from build123d import *

# Parameters (mm, degrees)
F0_W      = 59
F0_H      = 46
F1_DEPTH  = 32
F2_W      = 10
F2_H      = 6
F3_DEPTH  = 59
F4_W      = 33
F4_H      = 10
F5_DEPTH  = 23
F6_DEPTH  = 32
F8_DEPTH  = 26
F9_W      = 16
F9_H      = 12
F9_W_2    = 22
F10_DEPTH = 26
F12_DEPTH = 2
F13_R     = 2.5
F14_DEPTH = 25


with BuildPart() as f1:
    # F0 (on Top) → F1 (new body)
    with BuildSketch(Plane.XY):
        Rectangle(F0_W, F0_H)
    extrude(amount=F1_DEPTH)

    # F2 (on face) → F3 (cut)
    with BuildSketch(Plane.YZ.offset(29.5)):
        with Locations((0, 3)):
            Rectangle(F2_W, F2_H)
    extrude(amount=-F3_DEPTH, mode=Mode.SUBTRACT)

    # F4 (on face) → F5 (cut)
    with BuildSketch(Plane.XY.offset(32)):
        with Locations((13, -18)):
            Rectangle(F4_W, F4_H)
        with Locations((13, 18)):
            Rectangle(F4_W, F4_H)
    extrude(amount=-F5_DEPTH, mode=Mode.SUBTRACT)

    # F4 (on face) → F6 (join)
    with BuildSketch(Plane.XY.offset(32)):
        Polygon((-42.5, -13), (-29.5, -23), (-29.5, 23), (-42.5, 13), align=None)
    extrude(amount=-F6_DEPTH)

    # F7 (on face) → F8 (cut)
    with BuildSketch(Plane.XZ.offset(13)):
        Polygon((29.5, 25), (29.5, 32), (22.5, 32), align=None)
    extrude(amount=-F8_DEPTH, mode=Mode.SUBTRACT)

    # F9 (on face) → F10 (cut)
    with BuildSketch(Plane.XY.offset(32)):
        with Locations((4.5, 0)):
            Rectangle(F9_W, F9_H)
        with Locations((-14.5, 0)):
            Rectangle(F9_W_2, F9_H)
        with BuildLine():
            ThreePointArc((12.5, -6), (18.5, 0), (12.5, 6))
            Line((12.5, 6), (12.5, -6))
        make_face()
        with BuildLine():
            Line((-25.5, -6), (-25.5, 6))
            ThreePointArc((-25.5, 6), (-31.5, 0), (-25.5, -6))
        make_face()
    extrude(amount=-F10_DEPTH, mode=Mode.SUBTRACT)

    # F11 (on face) → F12 (cut)
    with BuildSketch(Plane.XY.offset(9)):
        Polygon((16.5, -15.719817), (12.979622, -13.734805), (9.500362, -15.791036), (9.54148, -19.832278), (13.061858, -21.817291), (16.541118, -19.76106), align=None)
        Polygon((13.061858, 21.817291), (9.54148, 19.832278), (9.500362, 15.791036), (12.979622, 13.734805), (16.5, 15.719817), (16.541118, 19.76106), align=None)
    extrude(amount=-F12_DEPTH, mode=Mode.SUBTRACT)

    # F13 (on face) → F14 (cut)
    with BuildSketch(Plane.XY.offset(7)):
        with BuildLine():
            ThreePointArc((15.52074, -17.776048), (14.779491, -15.999311), (12.995305, -15.276177))
            Line((12.995305, -15.276177), (13.046175, -20.275918))
            ThreePointArc((13.046175, -20.275918), (14.797477, -19.534799), (15.52074, -17.776048))
        make_face()
        with BuildLine():
            Line((13.046175, -20.275918), (12.995305, -15.276177))
            ThreePointArc((12.995305, -15.276177), (10.52087, -17.801483), (13.046175, -20.275918))
        make_face()
        with Locations((13.02074, 17.776048)):
            Circle(F13_R)
    extrude(amount=-F14_DEPTH, mode=Mode.SUBTRACT)


solid = f1.part
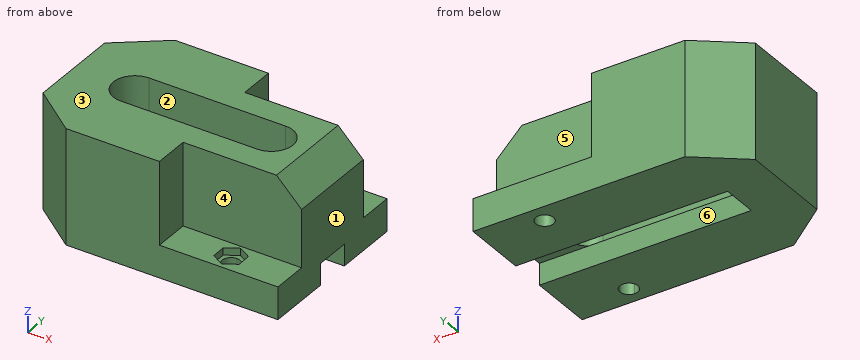
Check sheet for the modelled part. Datum: model origin and axes. Units: mm. Face numbers are marked on the shaded views. A direction names the side the tool comes from. Round coordinates to 2 decimals unless told otherwise and drop trailing zeros. Write each loop counter-clockwise with the first axis right and the second up, starting at its lowest first coordinate (ties: lowest second). Pieces come first, ordered by that corner, then holes. Notation, with made-up numbers: (58.5, 72.25) -> (67.5, 72.25) arc R3 cw to (67.5, 77.25) -> close; hole circle Ø10 at (33.5, -7). An arc over 180 degrees is marked (long way). Answer as CSV lines item,"result". Start each with the question number.
1) Section check D-D on z = 3. Enter the section's corners in (x, y).
2) Tool access check on the marked faces 4, 5 and 6. Record the directions out of +Z, -Z, +X, -X, +Y, -Y that give a thin tool (end or side, any length) a straight path to the whole face; none if there is none.
3) Section check B-B on z = 14. Enter the section's corners in (x, y).
4) Release check for a two-part mould opening along X. For the marked faces 1, 2 and 3 record: pulls with the +X half, pulls with the -X half, needs draft (parallel to the pull), parting line crosses it, or undercut.
5) Section check C-C on y = 0. Enter the section's corners in (x, z).
6) Section check A-A on x = -11.5. Enter the section's corners in (y, z).
7) Go/stop test with flat-tipped pins: P1, Ø3, axis at y = -2, z = 2.5, coming from the +X side; P2, Ø2, axis at x = 11.5, y = -19.5, coming from the +Z side; P3, Ø2, axis at x = 12, y = 17.5, coming from the +Z side; P4, Ø0.6, axis at x = -30, y = -1, coming from the +Z side. Record where each tip stops, or that it passes through.
8) Material ranges on line 1 (Y direction, x = -3, z = 13.5); line 2 (Y direction, x = -18.5, z = 18); line 3 (Z direction, x = 27, y = 15.5), recorded low to high. Write a range as from..to.
Found:
1,outline,"(-42.5, -13) -> (-29.5, -23) -> (29.5, -23) -> (29.5, -5) -> (-29.5, -5) -> (-29.5, 5) -> (29.5, 5) -> (29.5, 23) -> (-29.5, 23) -> (-42.5, 13) -> close; hole circle Ø5 at (13.02, 17.78); hole (13, -15.28) arc R2.5 ccw (long way) to (15.52, -17.78) arc R2.5 ccw to start"
2,face 4,"+Z, +X, -Y"
2,face 5,"+Z, +X, +Y"
2,face 6,"-Z, +X"
3,outline,"(-42.5, -13) -> (-29.5, -23) -> (-3.5, -23) -> (-3.5, -13) -> (29.5, -13) -> (29.5, 13) -> (-3.5, 13) -> (-3.5, 23) -> (-29.5, 23) -> (-42.5, 13) -> close; hole (-25.5, -6) -> (12.5, -6) arc R6 ccw to (12.5, 6) -> (-25.5, 6) arc R6 ccw to start"
4,face 1,"pulls with the +X half"
4,face 2,"undercut"
4,face 3,"needs draft"
5,outline,"(-42.5, 0) -> (-29.5, 0) -> (-29.5, 6) -> (-31.5, 6) -> (-31.5, 32) -> (-42.5, 32) -> close; (18.5, 6) -> (29.5, 6) -> (29.5, 25) -> (22.5, 32) -> (18.5, 32) -> close"
6,outline,"(-23, 0) -> (-5, 0) -> (-5, 6) -> (-6, 6) -> (-6, 32) -> (-23, 32) -> close; (5, 0) -> (23, 0) -> (23, 32) -> (6, 32) -> (6, 6) -> (5, 6) -> close"
7,P1,"stops at x = -29.5"
7,P2,"stops at z = 7"
7,P3,"passes through"
7,P4,"stops at z = 6"
8,line 1,"y = -13..-6, 6..13"
8,line 2,"y = -23..-6, 6..23"
8,line 3,"z = 0..9"
